Build history of the part. All positions in model axes, mm. Give positions to 0.01 mm unless a question says otherwise; leave off trailing zeros. Loops run counter-clockwise (first coordinate to the right, second up) from the corner with the lowest first, then second, coordinate; pieces in that order, holes last. Notation, with made-up numbers: (-9.75, 8.25) -> (43.25, 8.25) arc R19 ccw to (43.25, 16.25) -> close; hole circle Ø2 at (28.5, 31.5). An arc over 180 degrees is marked (long way). Answer as a JSON object with one key per item and string values. Group by question number.
Q1. Two-plate mould, pull along X, no slides. Class faces 1 (the cylindrical face through (-0.198, -0.07, 3.502)), 2 (the flat face through (13.5, 2.3, 12.5)), 3 (the flat face through (16.5, 0, 6)): pulls with the +X half, pulls with the -X half, needs draft (parallel to the pull), parting line crosses it, or undercut.
Q2. Band-saw the part on C-C, the plane x = -12.75. Write the cut outline in (y, z), plus the area to 4 significant figures.
Q3. Band-saw the part on D-D, the plane z = 7. Write the cut outline in (x, y), plus the area to 3 significant figures.
Q4. Drop a flat-ended pin along its axis: pin 1 (3 mm diameter, centred on x = 10.5, y = -3, fed in from -Z). Give the stop position or say it passes through.
Q5. Band-saw the part on B-B, the plane y = 0. Write the cut outline in (x, z).
Q6. Wall check: probe 1 along Y at (x, z) = (12.75, 5.25); probe 2 along X at (y, z) = (1.25, 0.75); probe 3 along X at (y, z) = (-2, 7). Give the ranges that are in metal, low to high. Write a range as from..to.
Q7. Band-saw the part on A-A, the plane z = 5. Write the cut outline in (x, y).
from build123d import *

# Parameters (mm, degrees)
F0_W     = 33
F0_H     = 10
F1_DEPTH = 12.5
F2_R     = 9
F3_DEPTH = 10
F4_R     = 2.25
F5_DEPTH = 12.5


with BuildPart() as f1:
    # F0 (on Top) → F1 (new body)
    with BuildSketch(Plane.XY):
        Rectangle(F0_W, F0_H)
    extrude(amount=F1_DEPTH)

    # F2 (on face) → F3 (cut)
    with BuildSketch(Plane.XZ.offset(5)):
        with Locations((0, 12.5)):
            Circle(F2_R)
    extrude(amount=-F3_DEPTH, mode=Mode.SUBTRACT)

    # F4 (on face) → F5 (cut)
    with BuildSketch(Plane.XY.offset(12.5)):
        with Locations((-12.75, 0)):
            Circle(F4_R)
        with Locations((12.75, 0)):
            Circle(F4_R)
    extrude(amount=-F5_DEPTH, mode=Mode.SUBTRACT)


solid = f1.part
Worked answers:
{
 "1": {"face 1": "undercut", "face 2": "needs draft", "face 3": "pulls with the +X half"},
 "2": {"outline": "(-5, 0) -> (-2.25, 0) -> (-2.25, 12.5) -> (-5, 12.5) -> close; (2.25, 0) -> (5, 0) -> (5, 12.5) -> (2.25, 12.5) -> close", "area": "68.75 mm2"},
 "3": {"outline": "(-16.5, -5) -> (-7.12, -5) -> (-7.12, 5) -> (-16.5, 5) -> close; (7.12, -5) -> (16.5, -5) -> (16.5, 5) -> (7.12, 5) -> close; hole circle Ø4.5 at (-12.75, 0); hole circle Ø4.5 at (12.75, 0)", "area": "156 mm2"},
 "4": {"pin 1": "z = 0"},
 "5": {"outline": "(-16.5, 0) -> (-15, 0) -> (-15, 12.5) -> (-16.5, 12.5) -> close; (-10.5, 0) -> (10.5, 0) -> (10.5, 12.5) -> (9, 12.5) arc R9 cw to (-9, 12.5) -> (-10.5, 12.5) -> close; (15, 0) -> (16.5, 0) -> (16.5, 12.5) -> (15, 12.5) -> close"},
 "6": {"probe 1": "-5..-2.25, 2.25..5", "probe 2": "-16.5..-14.62, -10.88..10.88, 14.62..16.5", "probe 3": "-16.5..-13.78, -11.72..-7.12, 7.12..11.72, 13.78..16.5"},
 "7": {"outline": "(-16.5, -5) -> (-4.97, -5) -> (-4.97, 5) -> (-16.5, 5) -> close; (4.97, -5) -> (16.5, -5) -> (16.5, 5) -> (4.97, 5) -> close; hole circle Ø4.5 at (-12.75, 0); hole circle Ø4.5 at (12.75, 0)"}
}
